```python
from build123d import *

# Parameters (mm, degrees)
SKETCH_1_R      = 1.65
SKETCH_1_R_2    = 1.6
EXTRUDE_1_DEPTH = 3
FILLET_2_R      = 10
FILLET_3_R      = 3


with BuildPart() as part:
    # 草图1 → 凸台-拉伸1 (new body)
    with BuildSketch(Plane.XY):
        with BuildLine():
            Line((-5.5, 2.397915762), (-8, -78.319172682))
            ThreePointArc((-8, -78.319172682), (0, -113.5), (8, -78.319172682))
            Line((8, -78.319172682), (5.5, 2.397915762))
            ThreePointArc((5.5, 2.397915762), (0, 6), (-5.5, 2.397915762))
        make_face()
        Circle(SKETCH_1_R, mode=Mode.SUBTRACT)
        with Locations((0, -95)):
            Circle(SKETCH_1_R_2, mode=Mode.SUBTRACT)
        with Locations((10.606601718, -84.393398282)):
            Circle(SKETCH_1_R_2, mode=Mode.SUBTRACT)
        with Locations((10.606601718, -105.606601718)):
            Circle(SKETCH_1_R_2, mode=Mode.SUBTRACT)
        with Locations((-10.606601718, -105.606601718)):
            Circle(SKETCH_1_R_2, mode=Mode.SUBTRACT)
        with Locations((-10.606601718, -84.393398282)):
            Circle(SKETCH_1_R_2, mode=Mode.SUBTRACT)
        with BuildLine():
            Line((-4.498993554, -64.390563515), (-4.79259564, -73.870045737))
            ThreePointArc((-4.79259564, -73.870045737), (0.155319711, -73.333901691), (5.095039914, -73.940928121))
            Line((5.095039914, -73.940928121), (4.799242432, -64.390563515))
            Line((4.799242432, -64.390563515), (-4.498993554, -64.390563515))
        make_face(mode=Mode.SUBTRACT)
        with BuildLine():
            ThreePointArc((6.933102995, -86.096444908), (0.107633433, -83.715957043), (-6.762002909, -85.965813425))
            ThreePointArc((-6.762002909, -85.965813425), (-7.121329366, -88.463845995), (-4.623296795, -88.823172453))
            ThreePointArc((-4.623296795, -88.823172453), (0.073590815, -87.284907246), (4.740280844, -88.912487427))
            ThreePointArc((4.740280844, -88.912487427), (7.244713179, -88.600877243), (6.933102995, -86.096444908))
        make_face(mode=Mode.SUBTRACT)
        with BuildLine():
            ThreePointArc((4.244153397, -105.456020867), (9.718451142, -100.735234766), (11.204836531, -93.661026988))
            ThreePointArc((11.204836531, -93.661026988), (9.221140094, -92.100824863), (7.660937969, -94.0845213))
            ThreePointArc((7.660937969, -94.0845213), (6.64467091, -98.921277892), (2.901800112, -102.148959919))
            ThreePointArc((2.901800112, -102.148959919), (1.91944628, -104.473667035), (4.244153397, -105.456020867))
        make_face(mode=Mode.SUBTRACT)
        with BuildLine():
            ThreePointArc((-11.177256391, -93.447534226), (-9.826084575, -100.548808191), (-4.442833622, -105.373159587))
            ThreePointArc((-4.442833622, -105.373159587), (-2.099810728, -104.435329142), (-3.037641173, -102.092306248))
            ThreePointArc((-3.037641173, -102.092306248), (-6.718261725, -98.793814861), (-7.642080956, -93.938552654))
            ThreePointArc((-7.642080956, -93.938552654), (-9.164159459, -91.925455722), (-11.177256391, -93.447534226))
        make_face(mode=Mode.SUBTRACT)
    extrude(amount=EXTRUDE_1_DEPTH)

    # 圆角2
    fillet_2_edges = [part.edges().sort_by_distance(p)[0] for p in [
        (8, -78.319172682, 1.5),
        (-8, -78.319172682, 1.5),
    ]]
    fillet(fillet_2_edges, radius=FILLET_2_R)

    # 圆角3
    fillet_3_edges = [part.edges().sort_by_distance(p)[0] for p in [
        (-4.79259564, -73.870045737, 1.5),
        (5.095039914, -73.940928121, 1.5),
        (4.799242432, -64.390563515, 1.5),
        (-4.498993554, -64.390563515, 1.5),
    ]]
    fillet(fillet_3_edges, radius=FILLET_3_R)


solid = part.part
```
CAD build for the part. Positions are in the model's coordinates, mm. Round coordinates to 2 decimals unless told otherwise and drop trailing zeros. Loops run counter-clockwise (first coordinate to the right, second up) from the corner with the lowest first, then second, coordinate; pieces in that order, holes last. Notation, with made-up numbers: M 74.5,-18.75 L 112.5,-18.75 A29 ccw 112.5,5.25 Z; hole C 21,36.5 d1. An arc over 180 degrees is marked long. Use a Markdown table: item, result. Add a question column.
(1) Cut at D-D (y = 0). Give the cut face in (x, z), and give its area (3 significant figures).
(2) Drill centre lines: line 1 (X direction, y = -95, z = 2.3); line 2 (Y direction, x = 0, z = 2.4); line 3 (Y direction, x = 0.5, z = 0.7). Where is each one in solid material? Low to high.
(3) Pull direction X, two halves, no side cores. Call faces 1 (the face through (-8.86, -77.18, 1.52)), 2 (the face through (-0.64, -113.49, 1.48)), 3 (the face through (-9.13, -91.93, 1.48)): +X half, -X half, draft (parallel to the pull), parting line (faces both ways), or undercut.
(4) Cut at B-B (x = 0). Give the cut face in (y, z), and give its area (3 significant figures).
(5) Cut at C-C (z = 2.15). State how many separate pieces and enclosed holes the cut face has, and give its area (3 significant figures).
(6) Flat gauge pin, fed straight in: pin 1 (3 mm diameter, centred on x = 0, y = -95, fed in from -Z). Where does the tip first touch, or does it go through?
(7) Cut at A-A (y = -98). Give the cut face in (x, z), and give its area (3 significant figures).
Geometry says:
| question | item | result |
|---|---|---|
| 1 | outline | M -5.57,0 L -1.65,0 L -1.65,3 L -5.57,3 Z; M 1.65,0 L 5.57,0 L 5.57,3 L 1.65,3 Z |
| 1 | area | 23.5 mm² |
| 2 | line 1 | x = -18.5 to -11.28, -7.72 to -1.6, 1.6 to 7.72, 11.28 to 18.5 |
| 2 | line 2 | y = -113.5 to -96.6, -93.4 to -87.28, -83.72 to -73.33, -64.39 to -1.65, 1.65 to 6 |
| 2 | line 3 | y = -113.49 to -96.52, -93.48 to -87.3, -83.73 to -73.34, -64.39 to -1.57, 1.57 to 5.98 |
| 3 | face 1 | -X half |
| 3 | face 2 | parting line |
| 3 | face 3 | undercut |
| 4 | outline | M -113.5,0 L -96.6,0 L -96.6,3 L -113.5,3 Z; M -93.4,0 L -87.28,0 L -87.28,3 L -93.4,3 Z; M -83.72,0 L -73.33,0 L -73.33,3 L -83.72,3 Z; M -64.39,0 L -1.65,0 L -1.65,3 L -64.39,3 Z; M 1.65,0 L 6,0 L 6,3 L 1.65,3 Z |
| 4 | area | 301 mm² |
| 5 | separate pieces | 1 |
| 5 | enclosed holes | 10 |
| 5 | area | 1,890 mm² |
| 6 | pin 1 | passes through |
| 7 | outline | M -18.26,0 L -10.88,0 L -10.88,3 L -18.26,3 Z; M -7.11,0 L 7.11,0 L 7.11,3 L -7.11,3 Z; M 10.88,0 L 18.26,0 L 18.26,3 L 10.88,3 Z |
| 7 | area | 86.9 mm² |
